Can you work these out from the model? Positions are in its coordinate system, mm. A direction names the side the tool comes from. Coordinates: 2 decimals unless noted, no trailing zeros. Order: outer loops, then holes, each group sorted by start corner. A loop starts at its lowest first (then second) coordinate and runs counter-clockwise, first axis right, second up. Notation, with made-up numbers: (38.5, 68.5) - (46.5, 68.5) arc R21 ccw to (46.5, 82.5) - close; hole circle Ø7 at (37.25, 77.5). An arc over 180 degrees is marked (long way). Return JSON: item names as keys, results as strings. Group by question number.
1) Which directions (+Z, -Z, +X, -X, +Y, -Y) give clear straight access to the entire face, cutting with the end or side of a thin tool? Please do faces 4 (the face through (53.748, -0.195, 10.162)), 5 (the face through (35.103, -47.205, 1.565)), 6 (the face through (51, -28, 3.175)).
2) If I drill on line 1 along Y through (x, z) = (0, 0.9); line 2 along X through (y, z) = (18, 15.25); line 3 along X through (y, z) = (-42.5, 18), over which ranges is the centre line in solid material (lowest first)?
3) If we mould it in two halves opening along Y, with no side actions, what happens to faces 1 (the face through (-38, 34, 19.05)), 2 (the face through (-0.2, 58.7, 1.6)), 3 (the face through (-13.77, -61.99, 1.31))? For each: pulls with the +Y half, pulls with the -Y half, needs draft (parallel to the pull), parting line crosses it, or undercut.
4) For pin 1 Ø2.5 at (x, y) = (-57.37, 18.64) entering from -Z; pin 2 Ø5 at (x, y) = (35.46, -48.8) entering from +Z (3 decimals); pin 3 Ø6 at (x, z) = (27, 4.5) entering from +Y; pin 4 Ø5 at (y, z) = (49, 8) entering from +X, each with a flat end and sliding along its axis, tell me the tip position at first contact or that it passes through.
5) Imagine slicing it at A-A (x = 0). Write out the boundary of the cut face in (y, z) (3 decimals).
```python
from build123d import *

# Parameters (mm, degrees)
F0_R      = 63.5
F1_DEPTH  = 3.175
F2_R      = 57.15
F3_DEPTH  = 58.7375
F4_R      = 50.8
F5_DEPTH  = 50.8
F6_R      = 1.6383
F7_DEPTH  = 3.175
F8_R      = 1.1303
F9_DEPTH  = 5.55625
F10_R     = 8.89
F11_REACH = 88.645717139
F12_R     = 0.508
F13_W     = 139.7
F13_H     = 50.8
F14_DEPTH = 63.5


with BuildPart() as f1:
    # F0 (on Top) → F1 (new body)
    with BuildSketch(Plane.XY):
        Circle(F0_R)
    extrude(amount=F1_DEPTH)

    # F2 (on Top) → F3 (join)
    with BuildSketch(Plane.XY):
        Circle(F2_R)
    extrude(amount=F3_DEPTH)

    # F4 (on face) → F5 (cut)
    with BuildSketch(Plane(origin=(0, 0, 0), x_dir=(1, 0, 0), z_dir=(0, 0, -1))):
        Circle(F4_R)
    extrude(amount=-F5_DEPTH, mode=Mode.SUBTRACT)

    # F6 (on face) → F7 (cut, through all)
    with BuildSketch(Plane(origin=(0, 0, 0), x_dir=(1, 0, 0), z_dir=(0, 0, -1))):
        with Locations((0, -60.325)):
            Circle(F6_R)
        with Locations((35.4581453445, -48.8039501857)):
            Circle(F6_R)
        with Locations((57.3724843455, -18.6414501857)):
            Circle(F6_R)
        with Locations((57.3724843455, 18.6414501857)):
            Circle(F6_R)
        with Locations((35.4581453445, 48.8039501857)):
            Circle(F6_R)
        with Locations((0, 60.325)):
            Circle(F6_R)
        with Locations((-35.4581453445, 48.8039501857)):
            Circle(F6_R)
        with Locations((-57.3724843455, 18.6414501857)):
            Circle(F6_R)
        with Locations((-57.3724843455, -18.6414501857)):
            Circle(F6_R)
        with Locations((-35.4581453445, -48.8039501857)):
            Circle(F6_R)
    extrude(amount=-F7_DEPTH, mode=Mode.SUBTRACT)

    # F8 (on face) → F9 (cut)
    with BuildSketch(Plane(origin=(0, 0, 50.8), x_dir=(1, 0, 0), z_dir=(0, 0, -1))):
        with Locations((31.115, -31.115)):
            Circle(F8_R)
        with Locations((-31.115, -31.115)):
            Circle(F8_R)
        with Locations((-31.115, 31.115)):
            Circle(F8_R)
        with Locations((31.115, 31.115)):
            Circle(F8_R)
        with Locations((31.115, 0)):
            Circle(F8_R)
        with Locations((-31.115, 0)):
            Circle(F8_R)
    extrude(amount=-F9_DEPTH, mode=Mode.SUBTRACT)

    f11_end = f1.faces().sort_by_distance((-57.15, 0, 30.95625))[0]
    # F10 (on Right) → F11 (cut, up to a face of the model that its end follows)
    with BuildSketch(Plane.YZ):
        with Locations((0, 19.05)):
            Circle(F10_R)
    f11_long = extrude(amount=F11_REACH, mode=Mode.PRIVATE)
    add(split(f11_long, bisect_by=f11_end, keep=Keep.BOTTOM, mode=Mode.PRIVATE), mode=Mode.SUBTRACT)

    # F12
    f12_edges = [f1.edges().sort_by_distance(p)[0] for p in [
        (-57.15, 0, 58.7375),
        (-63.5, 0, 3.175),
        (-57.15, 0, 3.175),
        (50.345599, 6.779427, 13.29922),
        (50.016076, -8.89, 19.051457),
    ]]
    fillet(f12_edges, radius=F12_R)

    # F13 (on Front) → F14 (cut, symmetric)
    with BuildSketch(Plane.XZ):
        with Locations((0, 44.45)):
            Rectangle(F13_W, F13_H)
    extrude(amount=F14_DEPTH, both=True, mode=Mode.SUBTRACT)


solid = f1.part
```
Calculated:
{
 "1": {"face 4": "+Z, +X", "face 5": "+Z, -Z", "face 6": "+Z"},
 "2": {"line 1": "-63.5 to -61.96, -58.69 to -50.8, 50.8 to 58.69, 61.96 to 63.5", "line 2": "-54.24 to -47.5, 47.5 to 54.24", "line 3": "-38.21 to -27.83, 27.83 to 38.21"},
 "3": {"face 1": "needs draft", "face 2": "undercut", "face 3": "parting line crosses it"},
 "4": {"pin 1": "through", "pin 2": "z = 3.175", "pin 3": "y = 58.55", "pin 4": "x = 33.22"},
 "5": {"outline": "(-63.5, 0) - (-61.963, 0) - (-61.963, 3.175) - (-62.992, 3.175) arc R0.508 ccw to (-63.5, 2.667) - close; (-58.687, 0) - (-50.8, 0) - (-50.8, 19.05) - (-57.15, 19.05) - (-57.15, 3.683) arc R0.508 cw to (-57.658, 3.175) - (-58.687, 3.175) - close; (50.8, 0) - (58.687, 0) - (58.687, 3.175) - (57.658, 3.175) arc R0.508 cw to (57.15, 3.683) - (57.15, 19.05) - (50.8, 19.05) - close; (61.963, 0) - (63.5, 0) - (63.5, 2.667) arc R0.508 ccw to (62.992, 3.175) - (61.963, 3.175) - close"}
}
